For this review, take the finished solid that the model builds, in its own axes (mm). Coordinates: 2 decimals unless noted, no trailing zeros. Loops run counter-clockwise (first coordinate to the right, second up) from the corner with the lowest first, then second, coordinate; pieces in that order, holes last. Notation, with made-up numbers: (-19.75, 39) -> (26.25, 39) arc R14 cw to (26.25, 61) -> close; hole circle Ø8 at (27.25, 37). An arc over 180 degrees is marked (long way). One line per item, written item: value.
Autodesk Inventor part; units mm, degrees
ref_plane "YZ Plane" through (0, 0, 0) normal (1, 0, 0) x (0, 1, 0)
ref_plane "XZ Plane" through (0, 0, 0) normal (0, 1, 0) x (-1, 0, 0)
ref_plane "XY Plane" through (0, 0, 0) normal (0, 0, 1) x (1, 0, 0)
sketch "Sketch1" plane through (0, 0, 0) normal (0, 0, 1) x (1, 0, 0)
  line L0 (0, 0) -> (101.5, 0)
  line L1 (101.5, 0) -> (101.5, -220)
  line L2 (101.5, -220) -> (0, -220)
  line L3 (0, -220) -> (0, 0)
  dimension "d0" = 101.5
  dimension "d1" = 220
extrude "Extrusion1" add sketch "Sketch1" along normal blind 1.8
sketch "Sketch2" plane through (0, 0, 1.8) normal (0, 0, 1) x (1, 0, 0)
  line L0 (0, 0) -> (0, -220)
  line L1 (101.5, -220) -> (101.5, 0)
  line L2 (0, 0) -> (101.5, 0)
  line L3 (101.5, 0) -> (101.5, -10)
  line L4 (101.5, -10) -> (0, -10)
  line L5 (0, -10) -> (0, 0)
  line L6 (50.75, -10) -> (140.75, -10)
  line L7 (140.75, -10) -> (140.75, -153.5958)
  line L8 (140.75, -153.5958) -> (50.75, -153.5958)
  line L9 (50.75, -153.5958) -> (50.75, -10)
  circle A0 centre (50.75, -153.5958) radius 2.5
  line L10 (50.75, -153.5958) -> (50.75, -173.5958)
  circle A1 centre (50.75, -173.5958) radius 2.5
  line L11 (50.75, -153.5958) -> (50.75, -133.5958)
  circle A2 centre (50.75, -163.5958) radius 2.5
  line L12 (101.5, 0) -> (0, 0)
  line L13 (0, -220) -> (101.5, -220)
  line L14 (0, 0) -> (101.5, -220)
  line L15 (101.5, -220) -> (50.75, -110)
  line L16 (50.75, -110) -> (87.135, -110)
  circle A3 centre (50.75, -66.4042) radius 2.5
  line L17 (50.75, -113.5958) -> (50.75, -46.4042)
  circle A4 centre (50.75, -46.4042) radius 2.5
  line L18 (50.75, -113.5958) -> (50.75, -86.4042)
  circle A5 centre (50.75, -56.4042) radius 2.5
  dimension "d4" = 10
  dimension "d5" = 90
  dimension "d6" = 5
  dimension "d7" = 20
  dimension "d8" = 20
  dimension "d11" = 5
extrude "Extrusion2" cut sketch "Sketch2" against normal blind 10 contours A1 | A2 L10 | L10 A2 | A4 L9 | L9 A4 | A3 L9 | L9 A3 | A0 L10 L8 | L8 L9 A0 | A5 L9 | L9 A5 | L9 L10 A0
sketch "Sketch3" plane through (0, 0, 1.8) normal (0, 0, 1) x (1, 0, 0)
  line L0 (0, -220) -> (101.5, -220)
  line L1 (0, -220) -> (3, -220)
  line L2 (3, -220) -> (3, -210)
  line L3 (3, -210) -> (0, -210)
  line L4 (0, -210) -> (0, -220)
  point P0 (0, 0)
  dimension "d14" = 3
  dimension "d15" = 10
extrude "Extrusion3" cut sketch "Sketch3" against normal blind 10
properties part number "7001_Aluminum_Chasis_Coil_Assembly_Separator_Tx_Filter_MPSv2_v1" material "Aluminum 6061"
1. Take a section at A-A, the plane x = 50.75. Give the boundary of the cut face in (y, z).
Return value:
outline: (-220, 0) -> (-176.1, 0) -> (-176.1, 1.8) -> (-220, 1.8) -> close; (-171.1, 0) -> (-166.1, 0) -> (-166.1, 1.8) -> (-171.1, 1.8) -> close; (-161.1, 0) -> (-156.1, 0) -> (-156.1, 1.8) -> (-161.1, 1.8) -> close; (-151.1, 0) -> (-68.9, 0) -> (-68.9, 1.8) -> (-151.1, 1.8) -> close; (-63.9, 0) -> (-58.9, 0) -> (-58.9, 1.8) -> (-63.9, 1.8) -> close; (-53.9, 0) -> (-48.9, 0) -> (-48.9, 1.8) -> (-53.9, 1.8) -> close; (-43.9, 0) -> (0, 0) -> (0, 1.8) -> (-43.9, 1.8) -> close
2. The part is to be moulded in two halves that separate along Y. For faces 1 (the flat face through (50, -108, 1.8)), 2 (the cylindrical face through (51.904, -155.814, 0.913)), say which applies: pulls with the +Y half, pulls with the -Y half, needs draft (parallel to the pull), parting line crosses it, or undercut.
Return value:
face 1: needs draft
face 2: undercut
3. To check wall thickness, follow probe 1 along X at (y, z) = (-173.5, 0.85); probe 2 along X at (y, z) = (-162, 1.1). State the ranges of each line that lie inside material, in increasing order. Write a range as from..to.
Return value:
probe 1: x = 0..48.25, 53.25..101.5
probe 2: x = 0..48.83, 52.67..101.5
4. Insertion check: pin 1 Ø0.9 at (y, z) = (-216, 1) entering from -X; pin 2 Ø0.5 at (x, z) = (2, 0.5) entering from -Y; pin 3 Ø4 at (x, y) = (50.75, -66.4) entering from +Z. Each pin has a flat end and moves straight along its axis. Give the tip position at first contact, or say it passes through.
Return value:
pin 1: stops at x = 3
pin 2: stops at y = -210
pin 3: passes through
